```python
from build123d import *

# Parameters (mm, degrees)
F0_R     = 5
F1_DEPTH = 129
F3_D     = 5
F3_DEPTH = 35
F3_TIP   = 1.5021515476
F5_D     = 5
F5_DEPTH = 35
F5_TIP   = 1.5021515476
F8_DEPTH = 8


# Not quite as in the source:
# - a pattern or mirror of a feature is missing from the dataset's text; its kind, count and spacing are read off the source's solid


with BuildPart() as f1:
    # F0 (on Front) → F1 (new body, symmetric)
    with BuildSketch(Plane.XZ):
        Circle(F0_R)
    extrude(amount=F1_DEPTH, both=True)

    # F3
    with Locations(Plane.XZ.offset(129)):
        with Locations((0, 0)):
            Hole(F3_D / 2, depth=F3_DEPTH)
            with Locations((0, 0, -(F3_DEPTH + F3_TIP / 2))):  # 118° drill point
                Cone(0, F3_D / 2, F3_TIP, mode=Mode.SUBTRACT)

    # F5
    with Locations(Plane(origin=(0, 129, 0), x_dir=(-1, 0, 0), z_dir=(0, 1, 0))):
        with Locations((0, 0)):
            Hole(F5_D / 2, depth=F5_DEPTH)
            with Locations((0, 0, -(F5_DEPTH + F5_TIP / 2))):  # 118° drill point
                Cone(0, F5_D / 2, F5_TIP, mode=Mode.SUBTRACT)

    # F7 (on offset) → F8 (cut)
    with BuildSketch(Plane.XZ.offset(104)):
        with BuildLine():
            Line((-4, -3), (-4, 3))
            ThreePointArc((-4, 3), (-5, 0), (-4, -3))
        make_face()
        with BuildLine():
            ThreePointArc((5, 0), (4.7434164903, 1.5811388301), (4, 3))
            Line((4, 3), (4, -3))
            ThreePointArc((4, -3), (4.7434164903, -1.5811388301), (5, 0))
        make_face()
    f8 = extrude(amount=-F8_DEPTH, mode=Mode.SUBTRACT)

    # F8_copies: F8 across plane
    add(f8.mirror(Plane.ZX), mode=Mode.SUBTRACT)


solid = f1.part
```
Geometry check sheet. Reference: the model listing, model coordinates, mm. A direction names the side the tool comes from. Coordinates: 2 decimals unless noted, no trailing zeros. Write each loop counter-clockwise with the first axis right and the second up, starting at its lowest first coordinate (ties: lowest second). Pieces come first, ordered by that corner, then holes. Notation, with made-up numbers: M 66,30 L 100,30 A18 cw 100,45 Z; hole C -39.5,88.25 d9. An arc over 180 degrees is marked long. Use one line per item in the form item = value. Start each with the question number.
1) Section check A-A on y = -50. Enter the section's corners in (x, z), and give its area (3 significant figures).
2) Set-up check for faces 1 (the cylindrical face through (-0.54, 111.26, -2.44)), 2 (the flat face through (-4, -100, 0)), 3 (the flat face through (4, -100, 0)), 4 (the flat face through (2, 129, -2)), 5 (the cylindrical face through (4.619, -1.806, -1.915)): record each of +Z, -Z, +X, -X, +Y, -Y from which the full face is reachable in a straight line by a thin tool's end or side.
3) Thickness scan on probe 1 along X at (y, z) = (109, 0); probe 2 along Z at (x, y) = (4, -86.5). Record the ranges inside material, lowest first. Write a range as from..to.
4) Release check for a two-part mould opening along Y. For faces 6 (the flat face through (2, -129, -2)), 7 (the cylindrical face through (0.54, -111.26, -2.44)), 8 (the flat face through (4, 100, 0)), 9 (the conical face through (0.094, 92.759, -0.424)) record: pulls with the +Y half, pulls with the -Y half, needs draft (parallel to the pull), parting line crosses it, or undercut.
5) Go/stop test with flat-tipped pins: pin 1 Ø2 at (y, z) = (62, 2) entering from -X; pin 2 Ø1.8 at (y, z) = (98.5, 1.5) entering from +X; pin 3 Ø1.8 at (y, z) = (-100, 0) entering from -X. Record where each tip stops, or that it passes through.
Responses:
q1.outline = C 0,0 d10
q1.area = 78.5 mm2
q2.face_1 = +Y
q2.face_2 = +Z, -Z, -X
q2.face_3 = +Z, -Z, +X
q2.face_4 = +Z, -Z, +X, -X, +Y
q2.face_5 = +Y, -Y
q3.probe_1 = -5..-2.5, 2.5..5
q3.probe_2 = -3..3
q4.face_6 = pulls with the -Y half
q4.face_7 = needs draft
q4.face_8 = undercut
q4.face_9 = pulls with the +Y half
q5.pin_1 = -4.9
q5.pin_2 = 4
q5.pin_3 = -4
